Geometry: final body of the model. Coordinates: model frame, mm. Round coordinates to 2 decimals unless told otherwise and drop trailing zeros. Order: outer loops, then holes, each group sorted by start corner. A loop starts at its lowest first (then second) coordinate and runs counter-clockwise, first axis right, second up. Notation, with made-up numbers: (-4.5, 48.25) -> (43.5, 48.25) arc R30 cw to (43.5, 75.25) -> close; hole circle Ø5 at (46.25, -18.75). An arc over 180 degrees is marked (long way). Put each result on its own line as item: value.
Autodesk Inventor part; units mm, degrees
ref_plane "YZ Plane" through (0, 0, 0) normal (1, 0, 0) x (0, 1, 0)
ref_plane "XZ Plane" through (0, 0, 0) normal (0, 1, 0) x (-1, 0, 0)
ref_plane "XY Plane" through (0, 0, 0) normal (0, 0, 1) x (1, 0, 0)
sketch "Sketch1" plane through (0, 0, 0) normal (0, 0, 1) x (1, 0, 0)
  line L0 (-35, -35) -> (35, -35)
  line L1 (35, -35) -> (35, 35)
  line L2 (35, 35) -> (-35, 35)
  line L3 (-35, 35) -> (-35, -35)
  line L4 (-35, -35) -> (35, 35) construction
  line L5 (35, -35) -> (-35, 35) construction
  line L6 (15.1, -15.1) -> (-15.1, -15.1)
  line L7 (-15.1, -15.1) -> (-15.1, 15.1)
  line L8 (-15.1, 15.1) -> (15.1, 15.1)
  line L9 (15.1, 15.1) -> (15.1, -15.1)
  line L10 (15.1, -15.1) -> (-15.1, 15.1) construction
  line L11 (-15.1, -15.1) -> (15.1, 15.1) construction
  point P0 (0, 0)
  dimension "d172" = 30.2
  dimension "d181" = 19.9
  dimension "d187" = 19.9
  dimension "d189" = 70
extrude "Plate5" add sketch "Sketch1" along normal blind 3
sketch "Sketch9" plane through (0, 0, 3) normal (0, 0, 1) x (1, 0, 0)
  circle A0 centre (26.5165, -26.5165) radius 2.75
  line L0 (26.5165, 26.5165) -> (-26.5165, 26.5165) construction
  line L1 (-26.5165, 26.5165) -> (-26.5165, -26.5165) construction
  line L2 (-26.5165, -26.5165) -> (26.5165, -26.5165) construction
  line L3 (26.5165, -26.5165) -> (26.5165, 26.5165) construction
  line L4 (26.5165, 26.5165) -> (-26.5165, -26.5165) construction
  line L5 (-26.5165, 26.5165) -> (26.5165, -26.5165) construction
  circle A1 centre (-26.5165, -26.5165) radius 2.75
  circle A2 centre (26.5165, 26.5165) radius 2.75
  circle A3 centre (-26.5165, 26.5165) radius 2.75
  circle A4 centre (0, 0) radius 37.5 construction
  line L6 (-15.1, -15.1) -> (-15.1, 15.1)
  line L7 (-15.1, 15.1) -> (15.1, 15.1)
  line L8 (15.1, 15.1) -> (15.1, -15.1)
  line L9 (15.1, -15.1) -> (-15.1, -15.1)
  line L10 (35, -35) -> (-35, -35)
  line L11 (35, 35) -> (35, -35)
  line L12 (-35, 35) -> (35, 35)
  line L13 (-35, -35) -> (-35, 35)
  line L14 (-15, 15) -> (15, 15) construction
  line L15 (15, 15) -> (15, -15) construction
  line L16 (15, -15) -> (-15, -15) construction
  line L17 (-15, -15) -> (-15, 15) construction
  line L18 (-15, -15) -> (15, 15) construction
  dimension "d188" = 75
  dimension "d174" = 5.5
  dimension "d184" = 30
  dimension "d185" = 30
  dimension "d186" = 16.2868
extrude "Cut2" cut sketch "Sketch9" against normal blind 3 contours A0 | A1 | A2 | A3
fillet "Corner Round1" radius 6 4 edges at (35, 35, 1.5) (-35, 35, 1.5) (-35, -35, 1.5) (35, -35, 1.5)
fillet "Corner Round2" radius 1 4 edges at (-15.1, 15.1, 1.5) (-15.1, -15.1, 1.5) (15.1, -15.1, 1.5) (15.1, 15.1, 1.5)
properties part number "ANP 1426 FDS Way FLANGE 2" material "Stainless Steel"
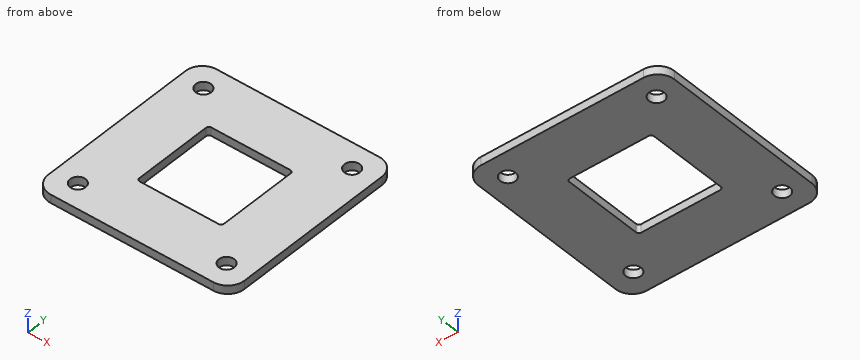
1. Cut plane C-C on y = -28. Return loops of the section in (x, z), and give its area (3 significant figures).
Ans:
outline: (-35, 0) -> (-28.83, 0) -> (-28.83, 3) -> (-35, 3) -> close; (-24.2, 0) -> (24.2, 0) -> (24.2, 3) -> (-24.2, 3) -> close; (28.83, 0) -> (35, 0) -> (35, 3) -> (28.83, 3) -> close
area: 182 mm²
2. Cut plane A-A on y = -5. Return loops of the section in (x, z).
Ans:
outline: (-35, 0) -> (-15.1, 0) -> (-15.1, 3) -> (-35, 3) -> close; (15.1, 0) -> (35, 0) -> (35, 3) -> (15.1, 3) -> close
3. Cut plane D-D on z = 1.85. Return loops of the section in (x, y).
Ans:
outline: (-35, -29) arc R6 ccw to (-29, -35) -> (29, -35) arc R6 ccw to (35, -29) -> (35, 29) arc R6 ccw to (29, 35) -> (-29, 35) arc R6 ccw to (-35, 29) -> close; hole circle Ø5.5 at (-26.52, -26.52); hole circle Ø5.5 at (-26.52, 26.52); hole (-15.1, -14.1) arc R1 ccw to (-14.1, -15.1) -> (14.1, -15.1) arc R1 ccw to (15.1, -14.1) -> (15.1, 14.1) arc R1 ccw to (14.1, 15.1) -> (-14.1, 15.1) arc R1 ccw to (-15.1, 14.1) -> close; hole circle Ø5.5 at (26.52, -26.52); hole circle Ø5.5 at (26.52, 26.52)
4. Material intervals for probe 1 along Y at (x, z) = (26.5, 1.5); probe 2 along X at (y, z) = (-9, 1.9); probe 3 along X at (y, z) = (29, 0.25), sorted ascending.
Ans:
probe 1: -35 to -29.27, -23.77 to 23.77, 29.27 to 35
probe 2: -35 to -15.1, 15.1 to 35
probe 3: -35 to -27.7, -25.34 to 25.34, 27.7 to 35
